Here's how the part is built. I have some questions about the finished solid (model axes, mm). A direction names the side the tool comes from. Coordinates: 2 decimals unless noted, no trailing zeros. Write each loop counter-clockwise with the first axis right and the second up, starting at its lowest first coordinate (ties: lowest second). Pieces come first, ordered by that corner, then holes. Notation, with made-up numbers: (44, -12) -> (49, -12) arc R17 ccw to (49, 19) -> close; hole circle Ø7 at (79, 73.25). An arc over 180 degrees is marked (long way). Use a Markdown table: item, result. Add a question column.
Item 1: Will these pins go through, and if not, where does the flat tip stop? pin 1 Ø5.5 at (x, y) = (-3.5, -3) entering from +Z; pin 2 Ø8 at (y, z) = (-5.5, 33) entering from +X; pin 3 Ø4 at (y, z) = (-13, 47) entering from +X; pin 4 Ø3 at (x, z) = (5.5, 49.5) entering from -Y.
Item 2: On a 3-axis mill with a long thin cutter (end or side, diameter ignored), from which of +Z, -Z, +X, -X, +Y, -Y can I reach the whole of each face in a straight line? I mean faces 1 (the flat face through (0, -28, 55)), 2 (the flat face through (27, 25, 30)), 3 (the flat face through (25, 0, 2)). Say none if no direction works.
Item 3: Imagine slicing it at C-C, the plane y = 0. Write out the boundary of the cut face in (x, z), and give its area (3 significant figures).
Item 4: Imagine slicing it at A-A, the plane z = 36. Write out the boundary of the cut face in (x, y), and give its area (3 significant figures).
Item 5: If I drill on line 1 along Y through (x, z) = (0, 26); line 2 along X through (y, z) = (-14, 2); line 3 along Z through (x, y) = (-7, 26), over which ranges is the centre line in solid material (lowest first)? Write a range as from..to.
Item 6: If we mould it in two halves opening along Z, with no side actions, what happens to faces 4 (the flat face through (0, -25, 2)), 5 (the flat face through (-25, -28, 30)), 6 (the flat face through (-25, 27, 30)), 7 (the flat face through (-27, 0, 60))? For each: pulls with the +Z half, pulls with the -Z half, needs draft (parallel to the pull), parting line crosses it, or undercut.
Item 7: Imagine slicing it at B-B, the plane x = 22. Write out the boundary of the cut face in (y, z).
```python
from build123d import *

# Parameters (mm, degrees)
F0_W     = 60
F0_H     = 60
F0_W_2   = 50
F0_H_2   = 50
F0_R     = 10
F0_R_2   = 9
F1_DEPTH = 2
F2_DEPTH = 60
F3_W     = 50
F3_H     = 50
F4_DEPTH = 60.001
F5_W     = 50
F5_H     = 50
F6_DEPTH = 60.001
F7_DEPTH = 60


with BuildPart() as f1:
    # F0 (on Top) → F1 (new body)
    with BuildSketch(Plane.XY):
        Rectangle(F0_W, F0_H)
        Rectangle(F0_W_2, F0_H_2, mode=Mode.SUBTRACT)
        Rectangle(F0_W_2, F0_H_2)
        Circle(F0_R, mode=Mode.SUBTRACT)
        Circle(F0_R)
        Circle(F0_R_2, mode=Mode.SUBTRACT)
        Circle(F0_R_2)
    extrude(amount=-F1_DEPTH)

    # F0 (on Top) → F2 (join)
    with BuildSketch(Plane.XY):
        Rectangle(F0_W, F0_H)
        Rectangle(F0_W_2, F0_H_2, mode=Mode.SUBTRACT)
    extrude(amount=F2_DEPTH)

    # F3 (on face) → F4 (cut, through all)
    with BuildSketch(Plane(origin=(-30, 0, 0), x_dir=(0, -1, 0), z_dir=(-1, 0, 0))):
        with Locations((0, 30)):
            Rectangle(F3_W, F3_H)
    extrude(amount=-F4_DEPTH, mode=Mode.SUBTRACT)

    # F5 (on face) → F6 (cut, through all)
    with BuildSketch(Plane.XZ.offset(30)):
        with Locations((0, 30)):
            Rectangle(F5_W, F5_H)
    extrude(amount=-F6_DEPTH, mode=Mode.SUBTRACT)

    # F0 (on Top) → F7 (join)
    with BuildSketch(Plane.XY):
        Circle(F0_R)
        Circle(F0_R_2, mode=Mode.SUBTRACT)
    extrude(amount=F7_DEPTH)


solid = f1.part
```
Ans:
| question | item | result |
|---|---|---|
| 1 | pin 1 | stops at z = 0 |
| 1 | pin 2 | stops at x = 9.89 |
| 1 | pin 3 | passes through |
| 1 | pin 4 | stops at y = -9.17 |
| 2 | face 1 | -Y |
| 2 | face 2 | +X, -X |
| 2 | face 3 | +Z |
| 3 | outline | (-30, -2) -> (30, -2) -> (30, 5) -> (25, 5) -> (25, 0) -> (10, 0) -> (10, 60) -> (9, 60) -> (9, 0) -> (-9, 0) -> (-9, 60) -> (-10, 60) -> (-10, 0) -> (-25, 0) -> (-25, 5) -> (-30, 5) -> close; (-30, 55) -> (-25, 55) -> (-25, 60) -> (-30, 60) -> close; (25, 55) -> (30, 55) -> (30, 60) -> (25, 60) -> close |
| 3 | area | 340 mm^2 |
| 4 | outline | (-30, -30) -> (-25, -30) -> (-25, -25) -> (-30, -25) -> close; (-30, 25) -> (-25, 25) -> (-25, 30) -> (-30, 30) -> close; circle Ø20 at (0, 0); (25, -30) -> (30, -30) -> (30, -25) -> (25, -25) -> close; (25, 25) -> (30, 25) -> (30, 30) -> (25, 30) -> close; hole circle Ø18 at (0, 0) |
| 4 | area | 160 mm^2 |
| 5 | line 1 | y = -10..-9, 9..10 |
| 5 | line 2 | x = -30..-25, 25..30 |
| 5 | line 3 | z = -2..5, 55..60 |
| 6 | face 4 | needs draft |
| 6 | face 5 | undercut |
| 6 | face 6 | undercut |
| 6 | face 7 | pulls with the +Z half |
| 7 | outline | (-30, -2) -> (30, -2) -> (30, 5) -> (25, 5) -> (25, 0) -> (-25, 0) -> (-25, 5) -> (-30, 5) -> close; (-30, 55) -> (-25, 55) -> (-25, 60) -> (-30, 60) -> close; (25, 55) -> (30, 55) -> (30, 60) -> (25, 60) -> close |
